from build123d import *

# Parameters (mm, degrees)
SKETCH1_R           = 11.1125
SKETCH1_R_2         = 2.4892
BOSS_EXTRUDE1_DEPTH = 3.175


with BuildPart() as part:
    # Sketch1 → Boss-Extrude1 (new body)
    with BuildSketch(Plane(origin=(0, 0, 0), x_dir=(1, 0, 0), z_dir=(0, 1, 0))):
        with BuildLine():
            Line((142.632381685, 111.984564783), (142.632381685, -40.415435217))
            ThreePointArc((142.632381685, -40.415435217), (116.6794163, -58.165823863), (106.68, -87.975962792))
            Line((106.68, -87.975962792), (106.68, -138.775962792))
            Line((106.68, -138.775962792), (96.52, -138.775962792))
            ThreePointArc((96.52, -138.775962792), (85.109838908, -106.248091666), (55.88, -87.975962792))
            Line((55.88, -87.975962792), (-55.88, -87.975962792))
            ThreePointArc((-55.88, -87.975962792), (-85.109838908, -106.248091666), (-96.52, -138.775962792))
            Line((-96.52, -138.775962792), (-106.68, -138.775962792))
            Line((-106.68, -138.775962792), (-106.68, -87.975962792))
            ThreePointArc((-106.68, -87.975962792), (-116.6794163, -58.165823863), (-142.632381685, -40.415435217))
            Line((-142.632381685, -40.415435217), (-142.632381685, 111.984564783))
            ThreePointArc((-142.632381685, 111.984564783), (-134.600001748, 137.62278551), (-108.918256202, 129.730673295))
            Line((-108.918256202, 129.730673295), (-31.75, -10.478375174))
            ThreePointArc((-31.75, -10.478375174), (0, -42.228375174), (31.75, -10.478375174))
            Line((31.75, -10.478375174), (108.918256202, 129.730673295))
            ThreePointArc((108.918256202, 129.730673295), (134.600001748, 137.62278551), (142.632381685, 111.984564783))
        make_face()
        with Locations(Location((-60.484532313, 2.221624826, 0), (0, 0, 270))):
            Circle(SKETCH1_R, mode=Mode.SUBTRACT)
        with Locations(Location((-125.726814921, 120.76547091, 0), (0, 0, 270))):
            Circle(SKETCH1_R, mode=Mode.SUBTRACT)
        with Locations(Location((125.726814921, 120.76547091, 0), (0, 0, 270))):
            Circle(SKETCH1_R, mode=Mode.SUBTRACT)
        with Locations(Location((-101.9175, -67.628375174, 0), (0, 0, 270))):
            Circle(SKETCH1_R_2, mode=Mode.SUBTRACT)
        with Locations(Location((60.484532313, 2.221624826, 0), (0, 0, 270))):
            Circle(SKETCH1_R, mode=Mode.SUBTRACT)
        with Locations(Location((-89.2175, -67.628375174, 0), (0, 0, 270))):
            Circle(SKETCH1_R_2, mode=Mode.SUBTRACT)
        with Locations(Location((-76.5175, -67.628375174, 0), (0, 0, 270))):
            Circle(SKETCH1_R_2, mode=Mode.SUBTRACT)
        with Locations(Location((-63.8175, -67.628375174, 0), (0, 0, 270))):
            Circle(SKETCH1_R_2, mode=Mode.SUBTRACT)
        with Locations(Location((-51.1175, -67.628375174, 0), (0, 0, 270))):
            Circle(SKETCH1_R_2, mode=Mode.SUBTRACT)
        with Locations(Location((-38.4175, -67.628375174, 0), (0, 0, 270))):
            Circle(SKETCH1_R_2, mode=Mode.SUBTRACT)
        with Locations(Location((-25.7175, -67.628375174, 0), (0, 0, 270))):
            Circle(SKETCH1_R_2, mode=Mode.SUBTRACT)
        with Locations(Location((-13.0175, -67.628375174, 0), (0, 0, 270))):
            Circle(SKETCH1_R_2, mode=Mode.SUBTRACT)
        with Locations(Location((-0.3175, -67.628375174, 0), (0, 0, 270))):
            Circle(SKETCH1_R_2, mode=Mode.SUBTRACT)
        with Locations(Location((12.3825, -67.628375174, 0), (0, 0, 270))):
            Circle(SKETCH1_R_2, mode=Mode.SUBTRACT)
        with Locations(Location((25.0825, -67.628375174, 0), (0, 0, 270))):
            Circle(SKETCH1_R_2, mode=Mode.SUBTRACT)
        with Locations(Location((37.7825, -67.628375174, 0), (0, 0, 270))):
            Circle(SKETCH1_R_2, mode=Mode.SUBTRACT)
        with Locations(Location((50.4825, -67.628375174, 0), (0, 0, 270))):
            Circle(SKETCH1_R_2, mode=Mode.SUBTRACT)
        with Locations(Location((63.1825, -67.628375174, 0), (0, 0, 270))):
            Circle(SKETCH1_R_2, mode=Mode.SUBTRACT)
        with Locations(Location((75.8825, -67.628375174, 0), (0, 0, 270))):
            Circle(SKETCH1_R_2, mode=Mode.SUBTRACT)
        with Locations(Location((88.5825, -67.628375174, 0), (0, 0, 270))):
            Circle(SKETCH1_R_2, mode=Mode.SUBTRACT)
        with Locations(Location((101.2825, -67.628375174, 0), (0, 0, 270))):
            Circle(SKETCH1_R_2, mode=Mode.SUBTRACT)
        with Locations(Location((-101.9175, -80.328375174, 0), (0, 0, 270))):
            Circle(SKETCH1_R_2, mode=Mode.SUBTRACT)
        with Locations(Location((-101.9175, -93.028375174, 0), (0, 0, 270))):
            Circle(SKETCH1_R_2, mode=Mode.SUBTRACT)
        with Locations(Location((-101.9175, -105.728375174, 0), (0, 0, 270))):
            Circle(SKETCH1_R_2, mode=Mode.SUBTRACT)
        with Locations(Location((-101.9175, -118.428375174, 0), (0, 0, 270))):
            Circle(SKETCH1_R_2, mode=Mode.SUBTRACT)
        with Locations(Location((-101.9175, -131.128375174, 0), (0, 0, 270))):
            Circle(SKETCH1_R_2, mode=Mode.SUBTRACT)
        with Locations(Location((101.2825, -80.328375174, 0), (0, 0, 270))):
            Circle(SKETCH1_R_2, mode=Mode.SUBTRACT)
        with Locations(Location((101.2825, -93.028375174, 0), (0, 0, 270))):
            Circle(SKETCH1_R_2, mode=Mode.SUBTRACT)
        with Locations(Location((101.2825, -105.728375174, 0), (0, 0, 270))):
            Circle(SKETCH1_R_2, mode=Mode.SUBTRACT)
        with Locations(Location((101.2825, -118.428375174, 0), (0, 0, 270))):
            Circle(SKETCH1_R_2, mode=Mode.SUBTRACT)
        with Locations(Location((101.2825, -131.128375174, 0), (0, 0, 270))):
            Circle(SKETCH1_R_2, mode=Mode.SUBTRACT)
        with Locations(Location((-106.68, -20.003375174, 0), (0, 0, 270))):
            Circle(SKETCH1_R, mode=Mode.SUBTRACT)
        with Locations(Location((106.68, -20.003375174, 0), (0, 0, 270))):
            Circle(SKETCH1_R, mode=Mode.SUBTRACT)
    extrude(amount=BOSS_EXTRUDE1_DEPTH)


solid = part.part
Design review of the part built by this model. Coordinates are the model's own, in mm. A direction names the side the tool comes from. Give positions to 0.01 mm unless a question says otherwise; leave off trailing zeros. Loops run counter-clockwise (first coordinate to the right, second up) from the corner with the lowest first, then second, coordinate; pieces in that order, holes last. Notation, with made-up numbers: (12, 38) - (40, 38) arc R14 ccw to (40, 45) - close; hole circle Ø4 at (81.25, 35.5). An arc over 180 degrees is marked (long way). Write item = value, one per line.
1) Take a section at A-A on y = 0.5. Count the separate pieces of the cut face and the enclosed holes in it, and give its area (3 significant figures).
Result sheet:
separate_pieces = 1
enclosed_holes = 33
area = 38,000 mm2
2) Tool access review of faces 1 (the face through (34, 0, 28)), 2 (the face through (-70.874, 1.565, -60.608)), 3 (the face through (-84.801, 1.565, 105.865)): name each direction out of +Z, -Z, +X, -X, +Y, -Y from which nothing blocks a thin tool from reaching the whole face with its end or side.
Result sheet:
face_1 = +Z, -Z, +X, -X, -Y
face_2 = -Z, +Y, -Y
face_3 = +Z, +Y, -Y
3) To check wall thickness, follow line 1 (Z direction, x = -52.5, y = 2.75); line 2 (X direction, y = 1.95, z = 120.5); line 3 (X direction, y = 2.6, z = 105). State the ranges of each line that lie inside material, in increasing order.
Result sheet:
line_1 = -27.22 to -9.95, 5.51 to 65.56, 69.7 to 87.98
line_2 = -106.68 to -103.3, -100.54 to -93.21, 93.21 to 99.9, 102.66 to 106.68
line_3 = -106.68 to -104.3, -99.54 to -84.08, 84.08 to 98.9, 103.66 to 106.68
4) Draft analysis for pull direction Z (two halves, no side actions). For faces 4 (the face through (-134.967, 1.565, -137.424)), 5 (the face through (34, 3.175, 28)), 6 (the face through (129.065, 1.565, -110.166)), state which applies: +Z half, -Z half, draft (parallel to the pull), parting line (faces both ways), or undercut.
Result sheet:
face_4 = parting line
face_5 = draft
face_6 = undercut
5) Take a section at B-B on x = 82.5. State the section outline as (y, z) points (3 decimals), and give its area (3 significant figures).
Result sheet:
outline = (0, -81.731) - (3.175, -81.731) - (3.175, 103.23) - (0, 103.23) - close
area = 587 mm2
6) Clearance check with flat-ended pins moving along their axes: pin 1 Ø4.5 at (x, z) = (88.58, 67.63) entering from -Y; pin 2 Ø1.6 at (x, y) = (-20, 1.5) entering from +Z; pin 3 Ø1.6 at (y, z) = (1, -59) entering from -X. State where each tip first meets the part, or that it passes through.
Result sheet:
pin_1 = through
pin_2 = 87.98
pin_3 = -142.63
